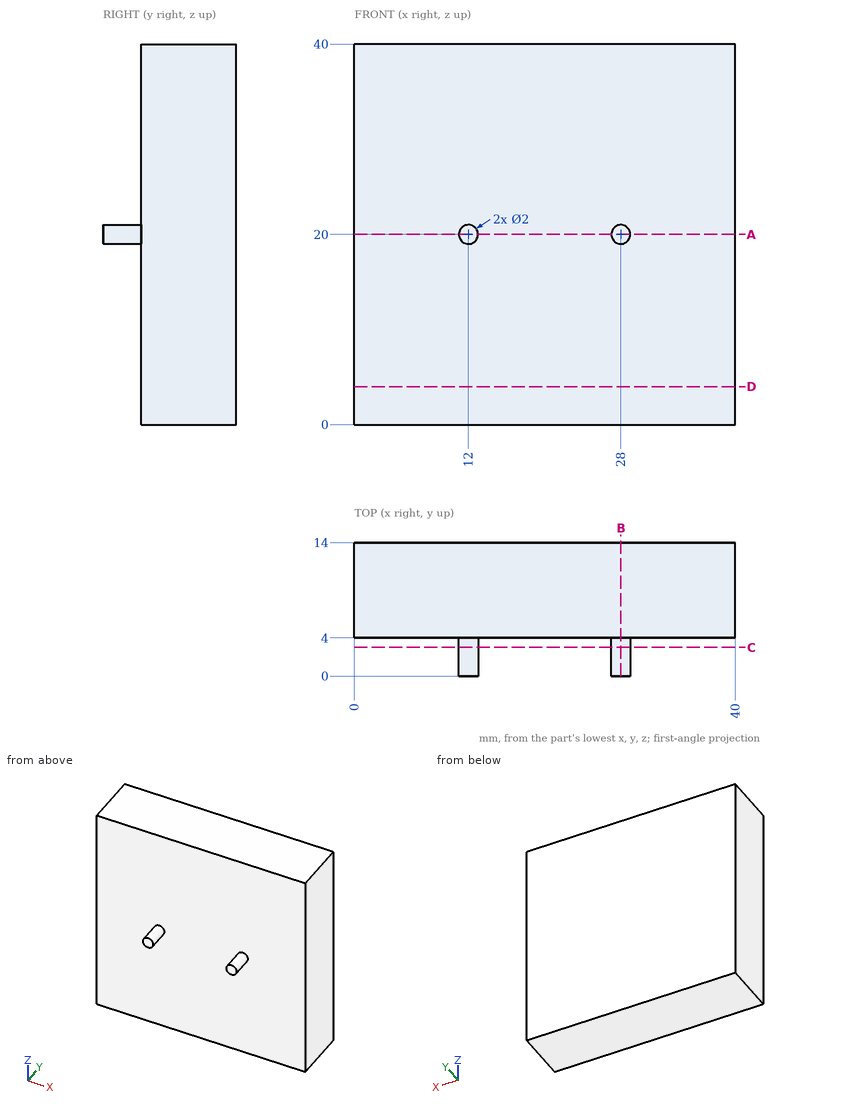
Can you work these out from the drawing? Everything is in mm from the part's minimum corner. Round coordinates to 2 decimals unless told otherwise and drop trailing zeros. Order: outer loops, then holes, each group sorted by start corner. A loop starts at its lowest first (then second) coordinate and runs counter-clockwise, first axis right, second up.
(1) If we section it at B-B (x = 28): Please give me the cut outline in (y, z), plus the area to 3 significant figures.
Results are:
outline: (0, 19) - (4, 19) - (4, 0) - (14, 0) - (14, 40) - (4, 40) - (4, 21) - (0, 21) - close
area: 408 mm2
(2) If I drill on L1, parallel to Y at x = 35, z = 3, over which ranges is the centre line in solid material (lowest first)?
Results are:
L1: y = 4 to 14
(3) If we section it at D-D (z = 4): Please give me the cut outline in (x, y).
Results are:
outline: (0, 4) - (40, 4) - (40, 14) - (0, 14) - close
(4) If we section it at A-A (z = 20): Please give me the cut outline in (x, y), plus the area to 3 significant figures.
Results are:
outline: (0, 4) - (11, 4) - (11, 0) - (13, 0) - (13, 4) - (27, 4) - (27, 0) - (29, 0) - (29, 4) - (40, 4) - (40, 14) - (0, 14) - close
area: 416 mm2
(5) I'm going to push flat-ended pins straight in: pin 1 (3 mm diameter, centred on x = 11, z = 12, fed in from -Y); pin 2 (5 mm diameter, centred on x = 15, y = 2.5, fed in from +Z). Where does each tip first touch, or does it pass through?
Results are:
pin 1: stops at y = 4
pin 2: stops at z = 40
(6) If we section it at C-C (y = 3): Please give me the cut outline in (x, z), plus the area to 3 significant figures.
Results are:
outline: circle Ø2 at (12, 20); circle Ø2 at (28, 20)
area: 6.28 mm2
